The listing builds one solid part. Answer for the finished solid, in the listing's coordinates (mm). Round coordinates to 2 decimals unless told otherwise and drop trailing zeros. Loops run counter-clockwise (first coordinate to the right, second up) from the corner with the lowest first, then second, coordinate; pieces in that order, holes last. Notation, with made-up numbers: M 23.5,-8.5 L 52.5,-8.5 A16 cw 52.5,-3.5 Z; hole C -4.5,46.5 d4. An arc over 180 degrees is marked long. Answer as a JSON object with one key per item and string values.
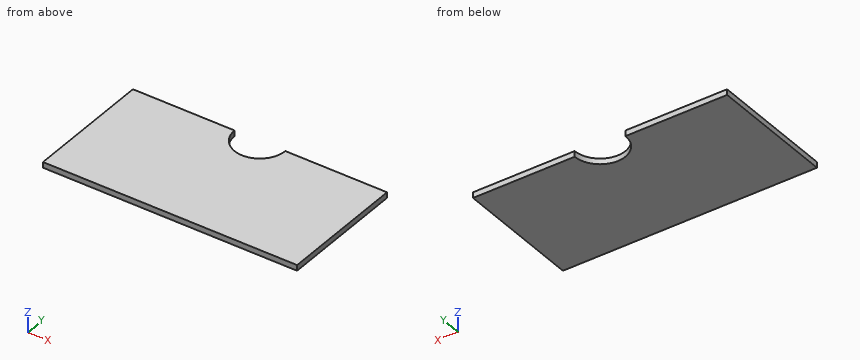
Autodesk Inventor part; units mm, degrees
ref_plane "YZ Plane" through (0, 0, 0) normal (1, 0, 0) x (0, 1, 0)
ref_plane "XZ Plane" through (0, 0, 0) normal (0, 1, 0) x (-1, 0, 0)
ref_plane "XY Plane" through (0, 0, 0) normal (0, 0, 1) x (1, 0, 0)
sketch "Sketch1" plane through (0, 0, 0) normal (0, 0, 1) x (1, 0, 0)
  line L0 (90, 0) -> (90, -90)
  line L1 (90, -90) -> (-90, -90)
  line L2 (-90, -90) -> (-90, 0)
  arc A0 (-18, 0) -> (18, 0) centre (0, 0) ccw
  line L3 (-90, 0) -> (-18, 0)
  line L4 (18, 0) -> (90, 0)
  dimension "d0" = 90
  dimension "d1" = 180
  dimension "d2" = 90
  dimension "d3" = 36
  dimension "d6" = 90
  dimension "d7" = 0
extrude "Extrusion1" add sketch "Sketch1" along normal blind 4
equation "\"BendRadius\" = Thickness"
equation "\"BendReliefWidth\" = Thickness"
equation "\"BendReliefDepth\" = 0.5 * Thickness"
equation "\"CornerReliefSize\" = 4 * Thickness"
equation "\"MinimumRemnant\" = 2 * Thickness"
equation "\"TransitionRadius\" = BendRadius"
equation "\"JacobiRadiusSize\" = BendRadius"
equation "\"GapSize\" = Thickness"
properties part number "Joint housing cover"
Item 1: The part is cut by section C-C (x = 0). Give the vertices of the cut face in (y, z).
Values follow:
{"outline": "M -90,0 L -18,0 L -18,4 L -90,4 Z"}
Item 2: The part is cut by section B-B (z = 1.55). Give the vertices of the cut face in (x, y).
Values follow:
{"outline": "M -90,-90 L 90,-90 L 90,0 L 18,0 A18 cw -18,0 L -90,0 Z"}
Item 3: The part is cut by section A-A (y = -10). Give the vertices of the cut face in (x, z).
Values follow:
{"outline": "M -90,0 L -14.97,0 L -14.97,4 L -90,4 Z; M 14.97,0 L 90,0 L 90,4 L 14.97,4 Z"}
Item 4: Straight lines are drawn through the part: line 1 (Y direction, x = 7, z = 2.85); line 2 (X direction, y = -8.5, z = 0.3); line 3 (X direction, y = -13, z = 0.7). For each, find the intervals that lie inside material, in ascending order.
Values follow:
{"line 1": "-90 to -16.58", "line 2": "-90 to -15.87, 15.87 to 90", "line 3": "-90 to -12.45, 12.45 to 90"}
